```python
from build123d import *

# Parameters (mm, degrees)
SKETCH1_W           = 80
SKETCH1_H           = 61
BOSS_EXTRUDE1_DEPTH = 12
SKETCH2_R           = 2.592161368
BOSS_EXTRUDE2_DEPTH = 12.5


with BuildPart() as part:
    # Sketch1 → Boss-Extrude1 (new body)
    with BuildSketch(Plane(origin=(0, 0, 0), x_dir=(1, 0, 0), z_dir=(0, 1, 0))):
        Rectangle(SKETCH1_W, SKETCH1_H)
    extrude(amount=BOSS_EXTRUDE1_DEPTH)

    # Sketch2 → Boss-Extrude2 (add)
    with BuildSketch(Plane.ZY.offset(40)):
        with Locations(Location((-15.567073505, 6.384900169, 0), (0, 0, 180))):
            Circle(SKETCH2_R)
        with Locations(Location((16.764540698, 6.384900169, 0), (0, 0, 180))):
            Circle(SKETCH2_R)
    extrude(amount=BOSS_EXTRUDE2_DEPTH)


solid = part.part
```
For this review, take the finished solid that the model builds, in its own axes (mm). A direction names the side the tool comes from. Coordinates: 2 decimals unless noted, no trailing zeros. Loops run counter-clockwise (first coordinate to the right, second up) from the corner with the lowest first, then second, coordinate; pieces in that order, holes last.
1. For faces 4 (the cylindrical face through (-46.16, 5.61, 14.29)), 5 (the flat face through (40, 6, 0)), list the 3-axis set-ups (+Z, -Z, +X, -X, +Y, -Y) from which the entire face can be reached by the end or side of a thin tool; tool diameter is ignored.
2. Add section C-C, the plane x = -42. Give the boundary of the cut face in (y, z).
3. Mouldability with a two-part tool opening along Z and no side actions: class faces 1 (the cylindrical face through (-46.16, 5.61, -18.04)), 2 (the flat face through (-1, 6, 30.5)), 3 (the flat face through (-1, 0, 0)) as +Z half, -Z half, draft (parallel to the pull), parting line (faces both ways), or undercut.
4. Add section D-D, the plane z = 22.5. Give the boundary of the cut face in (x, y).
5. Insertion check: P1, Ø6, axis at y = 6, z = -3, coming from the -X side; P2, Ø8, axis at x = 29.5, z = 16, coming from the -Y side. Each pin has a flat end and moves straight along its axis. Give the tip position at first contact, or say it passes through.
6. Add section A-A, the plane z = -16.5. Give the boundary of the cut face in (x, y), then the cut area to 3 significant figures.
7. For line 1 (X direction, y = 11.75, z = 17.5); line 2 (Y direction, x = -43, z = -13.5), list the stretches that pass through material, from the lowest coordinate up.
8. Add section B-B, the plane y = 4.75. Give the boundary of the cut face in (x, z), then the cut area to 3 significant figures.
Result:
1. face 4: -X
1. face 5: +Z, -Z, +X, +Y, -Y
2. outline: circle Ø5.18 at (6.38, -15.57); circle Ø5.18 at (6.38, 16.76)
3. face 1: undercut
3. face 2: +Z half
3. face 3: draft
4. outline: (-40, 0) - (40, 0) - (40, 12) - (-40, 12) - close
5. P1: stops at x = -40
5. P2: stops at y = 0
6. outline: (-52.5, 3.97) - (-40, 3.97) - (-40, 0) - (40, 0) - (40, 12) - (-40, 12) - (-40, 8.8) - (-52.5, 8.8) - close
6. area: 1,020 mm2
7. line 1: x = -40 to 40
7. line 2: y = 4.82 to 7.95
8. outline: (-52.5, -17.58) - (-40, -17.58) - (-40, -30.5) - (40, -30.5) - (40, 30.5) - (-40, 30.5) - (-40, 18.78) - (-52.5, 18.78) - (-52.5, 14.75) - (-40, 14.75) - (-40, -13.56) - (-52.5, -13.56) - close
8. area: 4,980 mm2
